Autodesk Fusion 360 part; units mm, degrees
sketch "Sketch1" plane through (0, 0, 0) normal (0, 1, 0) x (1, 0, 0)
  line L0 (-25.4646, 4.2269) -> (74.3574, 4.2269)
  line L1 (74.3574, 4.2269) -> (74.3574, -40.7311)
  line L2 (74.3574, -40.7311) -> (-25.4646, -40.7311)
  line L3 (-25.4646, -40.7311) -> (-25.4646, 4.2269)
  dimension "d1" = 99.822
  dimension "d2" = 44.958
extrude "Extrude1" add sketch "Sketch1" along normal blind 25.4
sketch "Sketch2" plane through (0, 0, 40.7311) normal (0, 0, 1) x (1, 0, 0)
  line L0 (-25.4646, 0) -> (74.3574, 0)
  line L1 (74.3574, 0) -> (74.3574, 25.4)
  line L2 (74.3574, 25.4) -> (-25.4646, 25.4)
  line L3 (-25.4646, 25.4) -> (-25.4646, 0)
  line L4 (-20.3846, 23.495) -> (69.2774, 23.495)
  line L5 (69.2774, 23.495) -> (69.2774, 0)
  line L6 (69.2774, 0) -> (-20.3846, 0)
  line L7 (-20.3846, 0) -> (-20.3846, 23.495)
  dimension "d5" = 5.08
  dimension "d6" = 5.08
  dimension "d7" = 1.905
extrude "Extrude2" cut sketch "Sketch2" against normal blind 66.04 contours L0 L4 L5 L6 L7
Could you check a few things on this model? Use its own coordinates, in mm. A direction names the side the tool comes from. Coordinates: 2 decimals unless noted, no trailing zeros. Write each loop counter-clockwise with the first axis right and the second up, starting at its lowest first coordinate (ties: lowest second). Pieces come first, ordered by that corner, then holes. Notation, with made-up numbers: (-27, 65) - (15, 65) arc R19 cw to (15, 72) - close; hole circle Ø1 at (26, 64). An arc over 180 degrees is marked (long way). Put each result on its own line as item: value. Start each with the question number.
Q1. Thinking about a two-plate mould opening in X: for faces 3 (the flat face through (-20.385, 12, 19)), 4 (the flat face through (-23, 0, 18)), 5 (the flat face through (74.357, 13, 18)), which applies, pulls with the +X half, pulls with the -X half, needs draft (parallel to the pull), parting line crosses it, or undercut?
Q2. I want a section at A-A on y = 10.75. Write out the boundary of the cut face in (x, z).
Q3. Please list where these lines run through material, in increasing order: L1, parallel to X at y = 3.5, z = 32.5; L2, parallel to Y at x = 6.5, z = 16 (3 decimals).
Q4. Which directions (+Z, -Z, +X, -X, +Y, -Y) give clear straight access to the entire face, cutting with the end or side of a thin tool? Please do faces 1 (the flat face through (24, 23.495, 19)), 2 (the flat face through (72, 0, 18)).
Q5. I want a section at B-B on z = 20. Write out the boundary of the cut face in (x, y) (3 decimals), plus the area to 3 significant figures.
Q6. I want a section at C-C on x = 48. Write out the boundary of the cut face in (y, z) (3 decimals).
Checks:
1. face 3: undercut
1. face 4: needs draft
1. face 5: pulls with the +X half
2. outline: (-25.46, -4.23) - (-20.38, -4.23) - (-20.38, 40.73) - (-25.46, 40.73) - close; (69.28, -4.23) - (74.36, -4.23) - (74.36, 40.73) - (69.28, 40.73) - close
3. L1: -25.46 to -20.38, 69.28 to 74.36
3. L2: 23.495 to 25.4
4. face 1: +Z, -Z, -Y
4. face 2: +Z, -Z, +X, -X, -Y
5. outline: (-25.465, 0) - (-20.385, 0) - (-20.385, 23.495) - (69.277, 23.495) - (69.277, 0) - (74.357, 0) - (74.357, 25.4) - (-25.465, 25.4) - close
5. area: 429 mm²
6. outline: (23.495, -4.227) - (25.4, -4.227) - (25.4, 40.731) - (23.495, 40.731) - close
